Geometry: final body of the model. Coordinates: model frame, mm. Give positions to 0.01 mm unless a question says otherwise; leave off trailing zeros. Order: outer loops, then holes, each group sorted by start corner. A loop starts at its lowest first (then second) coordinate and runs counter-clockwise, first axis right, second up. Notation, with made-up numbers: (54, 59.25) -> (92, 59.25) arc R28 ccw to (92, 89.25) -> close; hole circle Ø9 at (80, 19.5). An arc over 180 degrees is marked (long way). One line per question, with ' | ' between items.
from build123d import *

# Parameters (mm, degrees)
BOSS_EXTRUDE1_DEPTH = 4.7625
SKETCH2_R           = 14.2875
CUT_EXTRUDE1_DEPTH  = 127.195863524


with BuildPart() as part:
    # Sketch1 → Boss-Extrude1 (new body)
    with BuildSketch(Plane(origin=(0, 0, 0), x_dir=(1, 0, 0), z_dir=(0, 1, 0))):
        with BuildLine():
            Line((53.854446853, 73.373362576), (102.562489384, 58.945383065))
            Line((102.562489384, 58.945383065), (71.73313232, -45.132782137))
            Line((71.73313232, -45.132782137), (24.990181224, -31.286889228))
            ThreePointArc((24.990181224, -31.286889228), (23.967852385, -31.200180886), (22.994624733, -31.524992416))
            Line((22.994624733, -31.524992416), (-44.326137807, -70.562582621))
            ThreePointArc((-44.326137807, -70.562582621), (-52.787800823, -69.037356261), (-51.262574464, -60.575693244))
            Line((-51.262574464, -60.575693244), (53.854446853, 73.373362576))
        make_face()
    extrude(amount=BOSS_EXTRUDE1_DEPTH)

    # Sketch2 → Cut-Extrude1 (cut, through all)
    with BuildSketch(Plane(origin=(0, 4.7625, 0), x_dir=(1, 0, 0), z_dir=(0, 1, 0))):
        with Locations(Location((67.804408175, 31.44842364, 0), (0, 0, 270))):
            Circle(SKETCH2_R)
    extrude(amount=-CUT_EXTRUDE1_DEPTH, mode=Mode.SUBTRACT)


solid = part.part
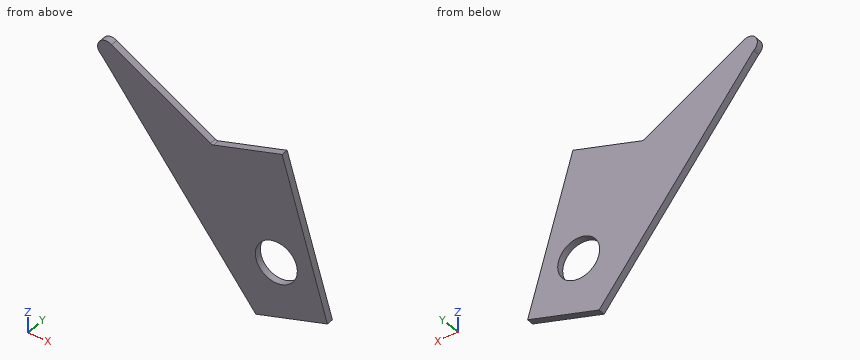
1) Section B-B on y = 1.4. Return loops of the section in (x, z) (1 decimal), plus the area to 3 significant figures.
Check result:
outline: (-51.3, 60.6) -> (53.9, -73.4) -> (102.6, -58.9) -> (71.7, 45.1) -> (25, 31.3) arc R2.5 cw to (23, 31.5) -> (-44.3, 70.6) arc R6.1 ccw to start; hole circle Ø28.6 at (67.8, -31.4) | area: 8,840 mm^2
2) Section C-C on z = -37. Return loops of the section in (x, y).
Check result:
outline: (25.31, 0) -> (54.64, 0) -> (54.64, 4.76) -> (25.31, 4.76) -> close; (80.97, 0) -> (96.06, 0) -> (96.06, 4.76) -> (80.97, 4.76) -> close
3) Contact query for flat-ended pins moving along their axis: pin 1 Ø1.5 at (y, z) = (4, 52) entering from +X; pin 2 Ø1.5 at (x, y) = (86, 3.5) entering from -Z; pin 3 Ø1.5 at (x, y) = (-1, 0.5) entering from +Z. Output: stop coordinate, or through.
Check result:
pin 1: stops at x = -11.02 | pin 2: stops at z = -64.07 | pin 3: stops at z = 45.87
4) Section A-A on x = 75. Return loops of the section in (y, z), plus the area to 3 significant figures.
Check result:
outline: (0, -67.11) -> (4.76, -67.11) -> (4.76, -43.79) -> (0, -43.79) -> close; (0, -19.11) -> (4.76, -19.11) -> (4.76, 34.1) -> (0, 34.1) -> close | area: 364 mm^2
5) Material intervals for probe 1 along Z at (x, y) = (57, 2.5); probe 2 along X at (y, z) = (2.5, -36); probe 3 along Z at (x, y) = (67.5, 2.75), sorted ascending. Write a range as from..to.
Check result:
probe 1: z = -72.44..-40.8, -22.1..40.77 | probe 2: x = 24.53..54.26, 81.35..95.77 | probe 3: z = -69.33..-45.73, -17.16..43.88
6) Section D-D on z = 13.5. Return loops of the section in (x, y).
Check result:
outline: (-14.32, 0) -> (81.1, 0) -> (81.1, 4.76) -> (-14.32, 4.76) -> close
